from build123d import *

# Parameters (mm, degrees)
SKETCH1_R               = 2.15
BOSS_EXTRUDE1_DEPTH     = 4
MIRROR2_COPY_1_SKETCH_R = 2.15
MIRROR2_COPY_1_DEPTH    = 4
SKETCH2_W               = 10.05
SKETCH2_H               = 20.05
CUT_EXTRUDE5_DEPTH      = 162.062099825


with BuildPart() as part:
    # Sketch1 → Boss-Extrude1 (new body)
    with BuildSketch(Plane(origin=(0, 0, 0), x_dir=(1, 0, 0), z_dir=(0, 1, 0))):
        with BuildLine():
            Line((135, -70), (0, -70))
            Line((0, -70), (0, 0))
            Line((0, 0), (145, 0))
            Line((145, 0), (145, -60))
            ThreePointArc((145, -60), (142.071067812, -67.071067812), (135, -70))
        make_face()
        with Locations(Location((135, -60, 0), (0, 0, 270))):
            Circle(SKETCH1_R, mode=Mode.SUBTRACT)
    boss_extrude1 = extrude(amount=BOSS_EXTRUDE1_DEPTH)

    # Mirror1: Boss-Extrude1 across plane
    add(boss_extrude1.mirror(Plane(origin=(0, 0, 0), x_dir=(0, 0, 1), z_dir=(1, 0, 0))))

    # Mirror2: Boss-Extrude1 across plane
    add(boss_extrude1.mirror(Plane.XY))

    # Mirror2 copy 1 sketch → Mirror2 copy 1 (add)
    with BuildSketch(Plane(origin=(0, 0, 0), x_dir=(-1, 0, 0), z_dir=(0, 1, 0))):
        with BuildLine():
            Line((135, -70), (0, -70))
            Line((0, -70), (0, 0))
            Line((0, 0), (145, 0))
            Line((145, 0), (145, -60))
            ThreePointArc((145, -60), (142.071067812, -67.071067812), (135, -70))
        make_face()
        with Locations(Location((135, -60, 0), (0, 0, 270))):
            Circle(MIRROR2_COPY_1_SKETCH_R, mode=Mode.SUBTRACT)
    extrude(amount=MIRROR2_COPY_1_DEPTH)

    # Sketch2 → Cut-Extrude5 (cut, through all)
    with BuildSketch(Plane(origin=(0, 4, 0), x_dir=(1, 0, 0), z_dir=(0, 1, 0))):
        with Locations((-0.025, -16.784138883)):
            Rectangle(SKETCH2_W, SKETCH2_H)
    extrude(amount=-CUT_EXTRUDE5_DEPTH, mode=Mode.SUBTRACT)


solid = part.part
For this review, take the finished solid that the model builds, in its own axes (mm). Round coordinates to 2 decimals unless told otherwise and drop trailing zeros. Order: outer loops, then holes, each group sorted by start corner. A loop starts at its lowest first (then second) coordinate and runs counter-clockwise, first axis right, second up. Notation, with made-up numbers: M 89.25,24.25 L 132.25,24.25 A20 ccw 132.25,28.25 Z; hole C 9,-20.5 d8. An arc over 180 degrees is marked long. Use a Markdown table: item, result. Add a question column.
Item 1: Add section A-A, the plane z = 10. Give the boundary of the cut face in (x, y).
Item 2: Insertion check: pin 1 (1 mm diameter, centred on x = -90.5, z = -16.5, fed in from -Y); pin 2 (2.5 mm diameter, centred on x = 135, z = 60, fed in from +Y). Each pin has a flat end and moves straight along its axis. Give the tip position at first contact, or say it passes through.
Item 3: To check wall thickness, follow line 1 along X through (y, z) = (2.3, 60); line 2 along Z through (x, y) = (-135, 1.65); line 3 along X through (y, z) = (1.9, 20). State the ranges of each line that lie inside material, in increasing order.
Geometry results:
| question | item | result |
|---|---|---|
| 1 | outline | M -145,0 L -5.05,0 L -5.05,4 L -145,4 Z; M 5,0 L 145,0 L 145,4 L 5,4 Z |
| 2 | pin 1 | stops at y = 0 |
| 2 | pin 2 | passes through |
| 3 | line 1 | x = -145 to -137.15, -132.85 to 132.85, 137.15 to 145 |
| 3 | line 2 | z = -70 to -62.15, -57.85 to 57.85, 62.15 to 70 |
| 3 | line 3 | x = -145 to -5.05, 5 to 145 |
